```python
from build123d import *

# Parameters (mm, degrees)
SKETCH2_W                 = 203.2
SKETCH2_H                 = 71.842048969
BOSS_EXTRUDE1_DEPTH       = 6.35
CUT_EXTRUDE1_DEPTH        = 203.2
CUT_EXTRUDE3_DEPTH        = 203.2
SKETCH7_R                 = 2.9
CUT_EXTRUDE4_DEPTH        = 6.35
LPATTERN1_COUNT           = 8
LPATTERN1_PITCH           = 21.166666667
LPATTERN2_COUNT           = 2
LPATTERN2_PITCH           = 15.875
LPATTERN2_COPY_1_SKETCH_R = 2.9
LPATTERN2_COPY_1_DEPTH    = 6.35
LPATTERN2_COPY_2_SKETCH_R = 2.9
LPATTERN2_COPY_2_DEPTH    = 6.35
LPATTERN2_COPY_3_SKETCH_R = 2.9
LPATTERN2_COPY_3_DEPTH    = 6.35
LPATTERN2_COPY_4_SKETCH_R = 2.9
LPATTERN2_COPY_4_DEPTH    = 6.35
LPATTERN2_COPY_5_SKETCH_R = 2.9
LPATTERN2_COPY_5_DEPTH    = 6.35
LPATTERN2_COPY_6_SKETCH_R = 2.9
LPATTERN2_COPY_6_DEPTH    = 6.35
LPATTERN2_COPY_7_SKETCH_R = 2.9
LPATTERN2_COPY_7_DEPTH    = 6.35
SKETCH8_R                 = 2.5
CUT_EXTRUDE5_DEPTH        = 6.35
LPATTERN3_COUNT           = 2
LPATTERN3_PITCH           = 15.875
SKETCH9_R                 = 3.375
CUT_EXTRUDE6_DEPTH        = 6.35
SKETCH12_R                = 3.175
CUT_EXTRUDE7_DEPTH        = 6.35


with BuildPart() as part:
    # Sketch2 → Boss-Extrude1 (new body)
    with BuildSketch(Plane.XY):
        with Locations((101.6, 35.921024485)):
            Rectangle(SKETCH2_W, SKETCH2_H)
    extrude(amount=BOSS_EXTRUDE1_DEPTH)

    # Sketch3 → Cut-Extrude1 (cut)
    with BuildSketch(Plane.ZY):
        Polygon((0, 0), (6.35, 0), (6.35, 6.35), align=None)
    extrude(amount=-CUT_EXTRUDE1_DEPTH, mode=Mode.SUBTRACT)

    # Sketch5 → Cut-Extrude3 (cut)
    with BuildSketch(Plane.ZY):
        Polygon((6.35, 71.842048969), (6.35, 65.492048969), (0, 71.842048969), align=None)
    extrude(amount=-CUT_EXTRUDE3_DEPTH, mode=Mode.SUBTRACT)

    # Sketch7 → Cut-Extrude4 (cut)
    with BuildSketch(Plane.XY.offset(6.35)):
        with Locations((15.875, 52.792048969)):
            Circle(SKETCH7_R)
    cut_extrude4 = extrude(amount=-CUT_EXTRUDE4_DEPTH, mode=Mode.SUBTRACT)

    # LPattern1: Cut-Extrude4 ×8
    with Locations(*[(i * LPATTERN1_PITCH, 0, 0) for i in range(1, LPATTERN1_COUNT)]):
        add(cut_extrude4, mode=Mode.SUBTRACT)

    # LPattern2: Cut-Extrude4 ×2
    with Locations(*[(0, -i * LPATTERN2_PITCH, 0) for i in range(1, LPATTERN2_COUNT)]):
        add(cut_extrude4, mode=Mode.SUBTRACT)

    # LPattern2 copy 1 sketch → LPattern2 copy 1 (cut)
    with BuildSketch(Plane(origin=(21.166666667, -15.875, 6.35), x_dir=(1, 0, 0), z_dir=(0, 0, 1))):
        with Locations((15.875, 52.792048969)):
            Circle(LPATTERN2_COPY_1_SKETCH_R)
    extrude(amount=-LPATTERN2_COPY_1_DEPTH, mode=Mode.SUBTRACT)

    # LPattern2 copy 2 sketch → LPattern2 copy 2 (cut)
    with BuildSketch(Plane(origin=(42.333333333, -15.875, 6.35), x_dir=(1, 0, 0), z_dir=(0, 0, 1))):
        with Locations((15.875, 52.792048969)):
            Circle(LPATTERN2_COPY_2_SKETCH_R)
    extrude(amount=-LPATTERN2_COPY_2_DEPTH, mode=Mode.SUBTRACT)

    # LPattern2 copy 3 sketch → LPattern2 copy 3 (cut)
    with BuildSketch(Plane(origin=(63.5, -15.875, 6.35), x_dir=(1, 0, 0), z_dir=(0, 0, 1))):
        with Locations((15.875, 52.792048969)):
            Circle(LPATTERN2_COPY_3_SKETCH_R)
    extrude(amount=-LPATTERN2_COPY_3_DEPTH, mode=Mode.SUBTRACT)

    # LPattern2 copy 4 sketch → LPattern2 copy 4 (cut)
    with BuildSketch(Plane(origin=(84.666666667, -15.875, 6.35), x_dir=(1, 0, 0), z_dir=(0, 0, 1))):
        with Locations((15.875, 52.792048969)):
            Circle(LPATTERN2_COPY_4_SKETCH_R)
    extrude(amount=-LPATTERN2_COPY_4_DEPTH, mode=Mode.SUBTRACT)

    # LPattern2 copy 5 sketch → LPattern2 copy 5 (cut)
    with BuildSketch(Plane(origin=(105.833333333, -15.875, 6.35), x_dir=(1, 0, 0), z_dir=(0, 0, 1))):
        with Locations((15.875, 52.792048969)):
            Circle(LPATTERN2_COPY_5_SKETCH_R)
    extrude(amount=-LPATTERN2_COPY_5_DEPTH, mode=Mode.SUBTRACT)

    # LPattern2 copy 6 sketch → LPattern2 copy 6 (cut)
    with BuildSketch(Plane(origin=(127, -15.875, 6.35), x_dir=(1, 0, 0), z_dir=(0, 0, 1))):
        with Locations((15.875, 52.792048969)):
            Circle(LPATTERN2_COPY_6_SKETCH_R)
    extrude(amount=-LPATTERN2_COPY_6_DEPTH, mode=Mode.SUBTRACT)

    # LPattern2 copy 7 sketch → LPattern2 copy 7 (cut)
    with BuildSketch(Plane(origin=(148.166666667, -15.875, 6.35), x_dir=(1, 0, 0), z_dir=(0, 0, 1))):
        with Locations((15.875, 52.792048969)):
            Circle(LPATTERN2_COPY_7_SKETCH_R)
    extrude(amount=-LPATTERN2_COPY_7_DEPTH, mode=Mode.SUBTRACT)

    # Sketch8 → Cut-Extrude5 (cut)
    with BuildSketch(Plane.XY.offset(6.35)):
        with Locations((187.325, 52.792048969)):
            Circle(SKETCH8_R)
    cut_extrude5 = extrude(amount=-CUT_EXTRUDE5_DEPTH, mode=Mode.SUBTRACT)

    # LPattern3: Cut-Extrude5 ×2
    with Locations(*[(0, -i * LPATTERN3_PITCH, 0) for i in range(1, LPATTERN3_COUNT)]):
        add(cut_extrude5, mode=Mode.SUBTRACT)

    # Sketch9 → Cut-Extrude6 (cut)
    with BuildSketch(Plane.XY.offset(6.35)):
        with Locations((187.325, 19.651113798)):
            Circle(SKETCH9_R)
    extrude(amount=-CUT_EXTRUDE6_DEPTH, mode=Mode.SUBTRACT)

    # Sketch12 → Cut-Extrude7 (cut)
    with BuildSketch(Plane.XY.offset(6.35)):
        with Locations((163.957, 18.464225693)):
            Circle(SKETCH12_R)
    extrude(amount=-CUT_EXTRUDE7_DEPTH, mode=Mode.SUBTRACT)


solid = part.part
```
Read the model definition and answer for the solid it produces. Units are mm, in the model's axes. Coordinates: 2 decimals unless noted, no trailing zeros. Write each loop counter-clockwise with the first axis right and the second up, starting at its lowest first coordinate (ties: lowest second). Pieces come first, ordered by that corner, then holes. Notation, with made-up numbers: (80.5, 9) - (115.5, 9) arc R27 cw to (115.5, 33) - close; hole circle Ø5 at (-11, 26.25). An arc over 180 degrees is marked (long way). Answer as a JSON object with one key per item and string values. Group by question number.
1. A cutting plane is placed at A-A (z = 1). Give the number of separate pieces and of enclosed holes in the cut face, plus the area to 3 significant figures.
2. Consider L1, parallel to Y at x = 164.5, z = 2; L2, parallel to Y at x = 78.5, z = 3.25; L3, parallel to X at y = 17.5, z = 6.25. Determine where each line is inside the solid, lowest interval first. Write a range as [from, to].
3. A cutting plane is placed at B-B (x = 23.5). Determine the outline of the cut face in (y, z).
4. The mould has two halves that part along Y. Classify faces 1 (the flat face through (100, 3, 3)), 2 (the flat face through (0, 35, 3)), 3 (the cylindrical face through (60.89, 35.81, 3.22)): +Y half, -Y half, draft (parallel to the pull), parting line (faces both ways), or undercut.
Worked out:
{
 "1": {"separate pieces": "1", "enclosed holes": "20", "area": "13,700 mm²"},
 "2": {"L1": "y = [2, 15.34], [21.59, 34.05], [39.78, 49.93], [55.66, 69.84]", "L2": "y = [3.25, 34.15], [39.68, 50.03], [55.56, 68.59]", "L3": "x = [0, 160.93], [166.98, 184.72], [189.93, 203.2]"},
 "3": {"outline": "(0, 0) - (71.84, 0) - (65.49, 6.35) - (6.35, 6.35) - close"},
 "4": {"face 1": "-Y half", "face 2": "draft", "face 3": "undercut"}
}
